from build123d import *

# Parameters (mm, degrees)
F2_R     = 7.5
F3_DEPTH = 33


with BuildPart() as f1:
    # F0 (on Right) → F1 (revolve)
    with BuildSketch(Plane.YZ):
        with BuildLine():
            Line((-60, 39), (-60, 31))
            Line((-60, 31), (-42, 29))
            Line((-42, 29), (-42, 26))
            Line((-42, 26), (0, 26))
            Line((0, 26), (0, 0))
            Line((0, 0), (30, 0))
            Line((30, 0), (30, 32))
            Line((30, 32), (33, 32))
            Line((33, 32), (33, 39))
            Line((33, 39), (0, 39))
            Line((0, 39), (-14.1321178182, 29.1045845728))
            ThreePointArc((-14.1321178182, 29.1045845728), (-19.3087430662, 28.7652906284), (-22, 33.2003447942))
            Line((-22, 33.2003447942), (-22, 45))
            Line((-22, 45), (-52, 45))
            Line((-52, 45), (-52, 39))
            Line((-52, 39), (-60, 39))
        make_face()
    revolve(axis=Axis((0, 15, 0), (0, -1, 0)))

    # F2 (on face) → F3 (join)
    with BuildSketch(Plane(origin=(0, 33, 0), x_dir=(-1, 0, 0), z_dir=(0, 1, 0))):
        with BuildLine():
            Line((20.2414907731, 58), (17.8346547716, 64.5517241379))
            ThreePointArc((17.8346547716, 64.5517241379), (0, 77), (-17.8346547716, 64.5517241379))
            Line((-17.8346547716, 64.5517241379), (-20.2414907731, 58))
            Line((-20.2414907731, 58), (-36.6079755837, 13.4482758621))
            ThreePointArc((-36.6079755837, 13.4482758621), (0, 39), (36.6079755837, 13.4482758621))
            Line((36.6079755837, 13.4482758621), (20.2414907731, 58))
        make_face()
        with Locations((0, 58)):
            Circle(F2_R, mode=Mode.SUBTRACT)
        with BuildLine():
            ThreePointArc((36.6079755837, -13.4482758621), (0, -39), (-36.6079755837, -13.4482758621))
            Line((-36.6079755837, -13.4482758621), (-20.2414907731, -58))
            Line((-20.2414907731, -58), (-17.8346547716, -64.5517241379))
            ThreePointArc((-17.8346547716, -64.5517241379), (0, -77), (17.8346547716, -64.5517241379))
            Line((17.8346547716, -64.5517241379), (20.2414907731, -58))
            Line((20.2414907731, -58), (36.6079755837, -13.4482758621))
        make_face()
        with Locations((0, -58)):
            Circle(F2_R, mode=Mode.SUBTRACT)
    extrude(amount=-F3_DEPTH)


solid = f1.part
Can you work these out from the model? Positions are in its coordinate system, mm. A direction names the side the tool comes from. Give positions to 0.01 mm unless a question says otherwise; leave off trailing zeros. Write each loop counter-clockwise with the first axis right and the second up, starting at its lowest first coordinate (ties: lowest second). Pieces come first, ordered by that corner, then holes. Notation, with made-up numbers: (45.25, 42) -> (52.25, 42) arc R17 cw to (52.25, 58) -> close; hole circle Ø4 at (-20.5, 79.5). An arc over 180 degrees is marked (long way). Answer as a JSON object with one key per item and string values. Group by question number.
Item 1: For faces 1 (the face through (30, -22, 17)), 2 (the face through (0, 30, 0)), 3 (the face through (15.821, -20.706, -20.633)), 4 (the face through (-39, 16, 0)), which set-ups out of +Z, -Z, +X, -X, +Y, -Y let a thin tool reach every point of the face, with its end or its side?
Item 2: Suppose I cut it at D-D (z = 0). Please give me the cut outline in (x, y), plus the area to 3 significant figures.
Item 3: I'm going to push flat-ended pins straight in: P1, Ø5, axis at x = -19, y = -47, coming from the -Z side; P2, Ø6, axis at x = 27.5, y = -35.5, coming from the -Z side; P3, Ø9, axis at x = 0, z = -58, coming from the +Y side; P4, Ø1.5, axis at y = -41, z = 38.5, coming from the +X side. Where does each tip first touch, or does it pass through?
Item 4: Suppose I cut it at C-C (y = -38). Please give me the cut outline in (x, z).
Item 5: We'd pull the mould along Y, two halves only. Please class faces 5 (the face through (31.24, 31.52, -6.94)), 6 (the face through (-37, -52, -14)), 7 (the face through (3, 0, -50)): +Y half, -Y half, draft (parallel to the pull), parting line (faces both ways), or undercut.
Item 6: Suppose I cut it at A-A (z = -53). Please give me the cut outline in (x, y), plus the area to 3 significant figures.
Item 7: Suppose I cut it at B-B (y = 13). Please give me the cut outline in (x, z).
Item 8: Please list where these lines run through material, in increasing order: line 1 (Y direction, x = 16.5, z = 17.5); line 2 (X direction, y = -14.5, z = 11); line 3 (Y direction, x = -16.5, z = 53). Write a range as [from, to].
Findings:
{
 "1": {"face 1": "none", "face 2": "+Y", "face 3": "-Y", "face 4": "-X, +Y"},
 "2": {"outline": "(-45, -52) -> (-39, -52) -> (-39, -60) -> (-31, -60) -> (-29, -42) -> (-26, -42) -> (-26, 0) -> (26, 0) -> (26, -42) -> (29, -42) -> (31, -60) -> (39, -60) -> (39, -52) -> (45, -52) -> (45, -22) -> (33.2, -22) arc R5 cw to (29.1, -14.13) -> (39, 0) -> (39, 33) -> (32, 33) -> (32, 30) -> (-32, 30) -> (-32, 33) -> (-39, 33) -> (-39, 0) -> (-29.1, -14.13) arc R5 cw to (-33.2, -22) -> (-45, -22) -> close", "area": "3,860 mm²"},
 "3": {"P1": "stops at z = -41.87", "P2": "stops at z = -37.75", "P3": "passes through", "P4": "stops at x = 24.49"},
 "4": {"outline": "circle Ø90 at (0, 0); hole circle Ø52 at (0, 0)"},
 "5": {"face 5": "draft", "face 6": "-Y half", "face 7": "undercut"},
 "6": {"outline": "(-22.08, 0) -> (-5.59, 0) -> (-5.59, 33) -> (-22.08, 33) -> close; (5.59, 0) -> (22.08, 0) -> (22.08, 33) -> (5.59, 33) -> close", "area": "1,090 mm²"},
 "7": {"outline": "(-36.61, -13.45) -> (-17.83, -64.55) arc R19 ccw to (17.83, -64.55) -> (36.61, -13.45) arc R39 ccw to (36.61, 13.45) -> (17.83, 64.55) arc R19 ccw to (-17.83, 64.55) -> (-36.61, 13.45) arc R39 ccw to start; hole circle Ø15 at (0, -58); hole circle Ø15 at (0, 58)"},
 "8": {"line 1": "y = [0, 30]", "line 2": "x = [-26.69, -23.56], [23.56, 26.69]", "line 3": "y = [0, 33]"}
}
